Autodesk Inventor part; units mm, degrees
ref_plane "YZ Plane" through (0, 0, 0) normal (1, 0, 0) x (0, 1, 0)
ref_plane "XZ Plane" through (0, 0, 0) normal (0, 1, 0) x (-1, 0, 0)
ref_plane "XY Plane" through (0, 0, 0) normal (0, 0, 1) x (1, 0, 0)
sketch "Sketch1" plane through (0, 0, 0) normal (1, 0, 0) x (0, 1, 0)
  line L0 (4.7302, 6.4139) -> (-20.6698, 6.4139)
  line L1 (-20.6698, 6.4139) -> (-20.6698, -18.9861)
  line L2 (-20.6698, -18.9861) -> (4.7302, -18.9861)
  line L3 (4.7302, -18.9861) -> (4.7302, 6.4139)
  line L4 (1.5552, 3.2389) -> (-17.4948, 3.2389)
  line L5 (-17.4948, 3.2389) -> (-17.4948, -15.8111)
  line L6 (-17.4948, -15.8111) -> (1.5552, -15.8111)
  line L7 (1.5552, -15.8111) -> (1.5552, 3.2389)
  point P0 (0, 0)
  dimension "d0" = 25.4
  dimension "d1" = 25.4
  dimension "d2" = 3.175
extrude "Extrusion1" add sketch "Sketch1" along normal blind 203.2
sketch "Sketch2" plane through (0, 4.7302, 6.4139) normal (0, 1, 0) x (1, 0, 0)
  line L0 (0, 3.175) -> (0, 22.225)
  circle A0 centre (25.4, 12.7) radius 3.175
  circle A1 centre (127, 12.7) radius 3.175
  point P0 (0, 6.4139)
  dimension "d6" = 6.35
  dimension "d8" = 6.35
extrude "Extrusion2" cut sketch "Sketch2" against normal blind 203.2
sketch "Sketch3" plane through (0, 4.7302, 6.4139) normal (0, 1, 0) x (1, 0, 0)
  line L0 (0, 25.4) -> (203.2, 25.4)
  line L1 (0, 22.225) -> (0, 3.175)
  circle A0 centre (66.802, 16.6589) radius 2.2987
  circle A1 centre (66.802, 3.1715) radius 2.2987
  circle A2 centre (50.8, 3.1715) radius 2.2987
  circle A3 centre (152.4, 16.6589) radius 2.2987
  circle A4 centre (152.4, 3.1715) radius 2.2987
  circle A5 centre (168.402, 3.1715) radius 2.2987
  circle A6 centre (168.402, 16.6589) radius 2.2987
  circle A7 centre (50.8, 16.6589) radius 2.2987
  point P0 (0, 6.4139)
extrude "Extrusion3" cut sketch "Sketch3" against normal blind 0.254
properties part number "Zero Twosday"
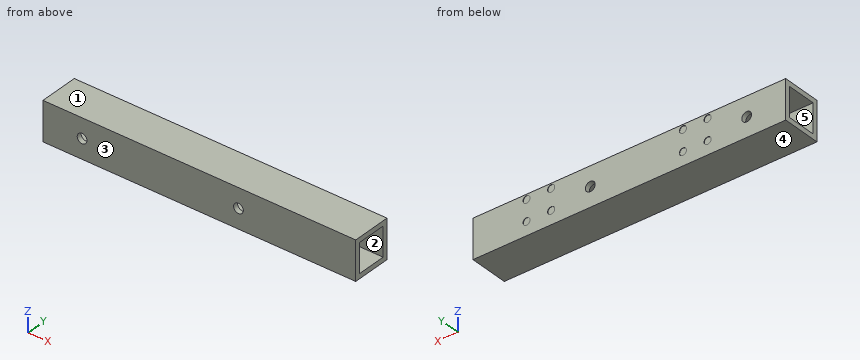
The model under review builds one solid part; all positions refer to its coordinate system, in mm. Face numbers are marked on the shaded views. A direction names the side the tool comes from. Round coordinates to 2 decimals unless told otherwise and drop trailing zeros. Write each loop counter-clockwise with the first axis right and the second up, starting at its lowest first coordinate (ties: lowest second). Pieces come first, ordered by that corner, then holes. Notation, with made-up numbers: (68.25, 13) -> (111.25, 13) arc R24 ccw to (111.25, 50) -> close; hole circle Ø4 at (39.25, -38). An arc over 180 degrees is marked (long way). Use CSV: the item, a comma, the result in double quotes.
Q1. Consider section C-C (x = 158.5). Give the boundary of the cut face in (y, z).
Checks:
outline,"(-20.67, -18.99) -> (4.73, -18.99) -> (4.73, 6.41) -> (-20.67, 6.41) -> close; hole (-17.49, -15.81) -> (1.56, -15.81) -> (1.56, 3.24) -> (-17.49, 3.24) -> close"
Q2. For pin 1 Ø1.4 at (x, z) = (167.5, 3.5) entering from +Y; pin 2 Ø5.5 at (x, z) = (25.4, -6.29) entering from -Y, all flat-tipped, find the tip position at first contact; note any pin that passes through.
Checks:
pin 1,"y = 4.48"
pin 2,"through"
Q3. To check wall thickness, follow probe 1 along Z at (x, y) = (152.4, 4.65); probe 2 along Y at (x, z) = (84, 0.75); probe 3 along Z at (x, y) = (80, 1.25). State the ranges of each line that lie inside material, in increasing order. Write a range as [from, to].
Checks:
probe 1,"[-18.99, -12.54], [-7.95, 0.94], [5.54, 6.41]"
probe 2,"[-20.67, -17.49], [1.56, 4.73]"
probe 3,"[-18.99, -15.81], [3.24, 6.41]"
Q4. Consider section B-B (x = 50.8). Give the boundary of the cut face in (y, z).
Checks:
outline,"(-20.67, -18.99) -> (4.73, -18.99) -> (4.73, -12.54) -> (4.48, -12.54) -> (4.48, -7.95) -> (4.73, -7.95) -> (4.73, 0.94) -> (4.48, 0.94) -> (4.48, 5.54) -> (4.73, 5.54) -> (4.73, 6.41) -> (-20.67, 6.41) -> close; hole (-17.49, -15.81) -> (1.56, -15.81) -> (1.56, 3.24) -> (-17.49, 3.24) -> close"
Q5. Mouldability with a two-part tool opening along Z and no side actions: class the marked faces 3, 4 and 5 as released by +Z, released by -Z, zero draft, split by the parting line, or undercut.
Checks:
face 3,"zero draft"
face 4,"released by -Z"
face 5,"undercut"
Q6. For the marked faces 1 and 2, list the 3-axis set-ups (+Z, -Z, +X, -X, +Y, -Y) from which the entire face can be reached by the end or side of a thin tool; tool diameter is ignored.
Checks:
face 1,"+Z, +X, -X, +Y, -Y"
face 2,"+X, -X"
Q7. Consider section A-A (x = 127). Give the boundary of the cut face in (y, z), then the cut area to 3 significant figures.
Checks:
outline,"(-20.67, -18.99) -> (4.73, -18.99) -> (4.73, -9.46) -> (1.56, -9.46) -> (1.56, -15.81) -> (-17.49, -15.81) -> (-17.49, -9.46) -> (-20.67, -9.46) -> close; (-20.67, -3.11) -> (-17.49, -3.11) -> (-17.49, 3.24) -> (1.56, 3.24) -> (1.56, -3.11) -> (4.73, -3.11) -> (4.73, 6.41) -> (-20.67, 6.41) -> close"
area,"242 mm²"
